Verification items for the finished model (mm, model axes). Face numbers are marked on the shaded views. A direction names the side the tool comes from. Round coordinates to 2 decimals unless told otherwise and drop trailing zeros. Order: outer loops, then holes, each group sorted by start corner. A loop starts at its lowest first (then second) coordinate and runs counter-clockwise, first axis right, second up. Notation, with made-up numbers: (33, 6.5) -> (47, 6.5) arc R32 cw to (47, 36.5) -> close; hole circle Ø9 at (2, -2). An arc over 180 degrees is marked (long way). Put each result on its own line as item: value.
from build123d import *

# Parameters (mm, degrees)
SKETCH1_W               = 35
SKETCH1_H               = 43
BOSS_EXTRUDE1_DEPTH     = 64
CUT_EXTRUDE1_DEPTH      = 77.04768241
CUT_EXTRUDE1_DEPTH_BACK = 77.04768241
CUT_EXTRUDE2_START      = -9
CUT_EXTRUDE2_DEPTH      = 9
CUT_EXTRUDE3_START      = -21
CUT_EXTRUDE3_DEPTH      = 21
SKETCH5_R               = 1.75
CUT_EXTRUDE4_DEPTH      = 21
CUT_EXTRUDE5_DEPTH      = 3
SKETCH7_R               = 1.75
CUT_EXTRUDE6_DEPTH      = 3
CUT_EXTRUDE7_DEPTH      = 2
SKETCH9_R               = 2.2
CUT_EXTRUDE8_DEPTH      = 78.474189407


# Read off the part's stored shape, not the designer's step: Cut-Extrude2, Cut-Extrude3
with BuildPart() as part:
    # Sketch1 → Boss-Extrude1 (new body)
    with BuildSketch(Plane.XY):
        Rectangle(SKETCH1_W, SKETCH1_H)
    extrude(amount=BOSS_EXTRUDE1_DEPTH)

    # Sketch2 → Cut-Extrude1 (cut, two sides: drawn at the far end of the back side and taken through both)
    with BuildSketch(Plane.ZY.offset(17.5).offset(-CUT_EXTRUDE1_DEPTH_BACK)):
        with BuildLine():
            Line((33.173885888, 11.5), (52, 11.5))
            Line((52, 11.5), (52, -10.5))
            Line((52, -10.5), (19.162446424, -10.499999995))
            add(Edge.make_bspline(
                [(19.162446424, -10.499999995), (20.832699675, -8.924322211), (23.191334331, -6.393604558), (26.156205176, -2.504954915), (28.325520723, 0.825456595), (30.873918563, 5.512287152), (32.363699443, 9.120198936), (33.173885888, 11.5)],
                knots=[0, 0, 0, 0, 0.261534973, 0.392989592, 0.556559744, 0.713681498, 1, 1, 1, 1], degree=3))
        make_face()
        with BuildLine():
            Line((0, -10.5), (0, 21.5))
            Line((0, 21.5), (24.5, 21.5))
            add(Edge.make_bspline(
                [(0, -10.5), (1.410254908, -9.794803553), (3.993077245, -8.365634948), (7.472082945, -6.021166025), (11.139491519, -3.071889035), (14.560754773, 0.394143772), (17.949614827, 4.871331165), (20.454917465, 9.23876326), (22.857889337, 14.900225374), (23.971477933, 18.909511405), (24.5, 21.5)],
                knots=[0, 0, 0, 0, 0.113112972, 0.211522862, 0.300551396, 0.450408793, 0.559434529, 0.702650577, 0.810275993, 1, 1, 1, 1], degree=3))
        make_face()
    extrude(amount=CUT_EXTRUDE1_DEPTH + CUT_EXTRUDE1_DEPTH_BACK, mode=Mode.SUBTRACT)

    # Cut-Extrude2 outline → Cut-Extrude2 (cut)
    with BuildSketch(Plane(origin=(17.5, 0, 0), x_dir=(0, 0, -1), z_dir=(1, 0, 0)).offset(CUT_EXTRUDE2_START)):
        with BuildLine():
            Line((-24.5, 21.5), (-59, 21.5))
            Line((-59, 21.5), (-59, -21.5))
            Line((-59, -21.5), (0, -21.5))
            Line((0, -21.5), (0, -10.5))
            add(Edge.make_bspline(
                [(0, -10.5), (-1.410254908, -9.794803553), (-3.993077245, -8.365634948), (-7.472082945, -6.021166025), (-11.139491519, -3.071889035), (-14.560754773, 0.394143772), (-17.949614827, 4.871331165), (-20.454917465, 9.23876326), (-22.857889337, 14.900225374), (-23.971477933, 18.909511405), (-24.5, 21.5)],
                knots=[0, 0, 0, 0, 0.113112972, 0.211522862, 0.300551396, 0.450408793, 0.559434529, 0.702650577, 0.810275993, 1, 1, 1, 1], degree=3))
        make_face()
        with BuildLine():
            Line((-52, 11.5), (-33.173885888, 11.5))
            add(Edge.make_bspline(
                [(-33.173885888, 11.5), (-32.363699443, 9.120198936), (-30.873918563, 5.512287152), (-28.325520723, 0.825456595), (-26.156205176, -2.504954915), (-23.191334331, -6.393604558), (-20.832699675, -8.924322211), (-19.162446424, -10.499999995)],
                knots=[0, 0, 0, 0, 0.286318502, 0.443440256, 0.607010408, 0.738465027, 1, 1, 1, 1], degree=3))
            Line((-19.162446424, -10.499999995), (-52, -10.5))
            Line((-52, -10.5), (-52, 11.5))
        make_face(mode=Mode.SUBTRACT)
    extrude(amount=CUT_EXTRUDE2_DEPTH, mode=Mode.SUBTRACT)

    # Cut-Extrude3 outline → Cut-Extrude3 (cut)
    with BuildSketch(Plane(origin=(8.5, 0, 0), x_dir=(0, 0, -1), z_dir=(1, 0, 0)).offset(CUT_EXTRUDE3_START)):
        with BuildLine():
            Line((-30.5, 16.5), (-59, 16.5))
            Line((-59, 16.5), (-59, -16.5))
            Line((-59, -16.5), (-51, -16.5))
            Line((-51, -16.5), (-51, -21.5))
            Line((-51, -21.5), (-10, -21.5))
            Line((-10, -21.5), (-10, -16.5))
            Line((-10, -16.5), (0, -16.5))
            Line((0, -16.5), (0, -10.5))
            add(Edge.make_bspline(
                [(0, -10.5), (-1.410254908, -9.794803553), (-3.993077245, -8.365634948), (-7.472082945, -6.021166025), (-11.139491519, -3.071889035), (-14.560754773, 0.394143772), (-17.949614827, 4.871331165), (-20.454917465, 9.23876326), (-22.857889337, 14.900225374), (-23.971477933, 18.909511405), (-24.5, 21.5)],
                knots=[0, 0, 0, 0, 0.113112972, 0.211522862, 0.300551396, 0.450408793, 0.559434529, 0.702650577, 0.810275993, 1, 1, 1, 1], degree=3))
            Line((-24.5, 21.5), (-30.5, 21.5))
            Line((-30.5, 21.5), (-30.5, 16.5))
        make_face()
        with BuildLine():
            Line((-52, 11.5), (-33.173885888, 11.5))
            add(Edge.make_bspline(
                [(-33.173885888, 11.5), (-32.363699443, 9.120198936), (-30.873918563, 5.512287152), (-28.325520723, 0.825456595), (-26.156205176, -2.504954915), (-23.191334331, -6.393604558), (-20.832699675, -8.924322211), (-19.162446424, -10.499999995)],
                knots=[0, 0, 0, 0, 0.286318502, 0.443440256, 0.607010408, 0.738465027, 1, 1, 1, 1], degree=3))
            Line((-19.162446424, -10.499999995), (-52, -10.5))
            Line((-52, -10.5), (-52, 11.5))
        make_face(mode=Mode.SUBTRACT)
    extrude(amount=CUT_EXTRUDE3_DEPTH, mode=Mode.SUBTRACT)

    # Sketch5 → Cut-Extrude4 (cut)
    with BuildSketch(Plane.XZ.offset(21.5)):
        with Locations(Location((3, 54.5, 0), (0, 0, 270))):
            Circle(SKETCH5_R)
        with Locations(Location((-7, 54.5, 0), (0, 0, 270))):
            Circle(SKETCH5_R)
        with Locations(Location((-7, 6.5, 0), (0, 0, 270))):
            Circle(SKETCH5_R)
        with Locations(Location((3, 6.5, 0), (0, 0, 270))):
            Circle(SKETCH5_R)
    extrude(amount=-CUT_EXTRUDE4_DEPTH, mode=Mode.SUBTRACT)

    # Sketch6 → Cut-Extrude5 (cut)
    with BuildSketch(Plane(origin=(0, 0, 59), x_dir=(-1, 0, 0), z_dir=(0, 0, -1))):
        Polygon((0.5, 5.095041723), (-2.7, 3.247520861), (-2.7, -0.447520861), (0.5, -2.295041723), (3.7, -0.447520861), (3.7, 3.247520861), align=None)
        Polygon((8.5, 5.095041723), (5.3, 3.247520861), (5.3, -0.447520861), (8.5, -2.295041723), (11.7, -0.447520861), (11.7, 3.247520861), align=None)
        Polygon((8.5, -6.904958277), (5.3, -8.752479139), (5.3, -12.447520861), (8.5, -14.295041723), (11.7, -12.447520861), (11.7, -8.752479139), align=None)
        Polygon((0.5, -6.904958277), (-2.7, -8.752479139), (-2.7, -12.447520861), (0.5, -14.295041723), (3.7, -12.447520861), (3.7, -8.752479139), align=None)
    extrude(amount=-CUT_EXTRUDE5_DEPTH, mode=Mode.SUBTRACT)

    # Sketch7 → Cut-Extrude6 (cut)
    with BuildSketch(Plane(origin=(0, 0, 62), x_dir=(-1, 0, 0), z_dir=(0, 0, -1))):
        with Locations((0.5, 1.4)):
            Circle(SKETCH7_R)
        with Locations((8.5, 1.4)):
            Circle(SKETCH7_R)
        with Locations((8.5, -10.6)):
            Circle(SKETCH7_R)
        with Locations((0.5, -10.6)):
            Circle(SKETCH7_R)
    extrude(amount=-CUT_EXTRUDE6_DEPTH, mode=Mode.SUBTRACT)

    # Sketch8 → Cut-Extrude7 (cut)
    with BuildSketch(Plane.XZ.offset(-16.5)):
        Polygon((1.7, 38.613804004), (1.7, 42.886195996), (-2, 45.022391992), (-5.7, 42.886195996), (-5.7, 38.613804004), (-2, 36.477608008), align=None)
    extrude(amount=-CUT_EXTRUDE7_DEPTH, mode=Mode.SUBTRACT)

    # Sketch9 → Cut-Extrude8 (cut, through all)
    with BuildSketch(Plane(origin=(0, 18.5, 0), x_dir=(-1, 0, 0), z_dir=(0, -1, 0))):
        with Locations(Location((2, -40.75, 0), (0, 0, 90))):
            Circle(SKETCH9_R)
    extrude(amount=-CUT_EXTRUDE8_DEPTH, mode=Mode.SUBTRACT)


solid = part.part
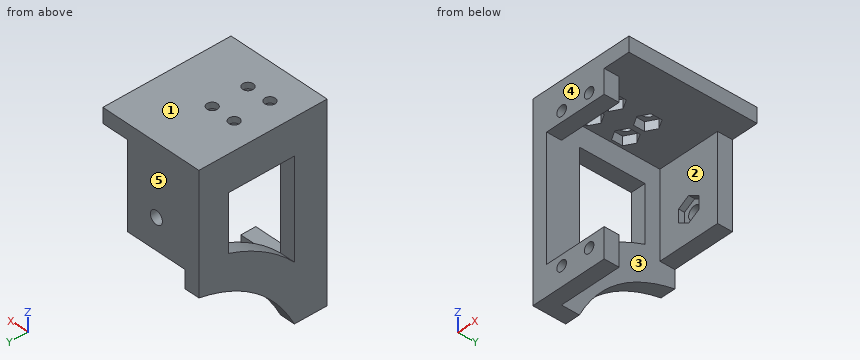
Item 1: Section check B-B on x = 4. Record the boundary of the cut face in (y, z), then the cut area to 3 significant figures.
Check sheet entries:
outline: (-21.5, 0) -> (-16.5, 0) -> (-16.5, 5.06) -> (-21.5, 5.06) -> close; (-21.5, 7.94) -> (-16.5, 7.94) -> (-16.5, 10) -> (-21.5, 10) -> close; (-21.5, 51) -> (-16.5, 51) -> (-16.5, 53.06) -> (-21.5, 53.06) -> close; (-21.5, 55.94) -> (-16.5, 55.94) -> (-16.5, 59) -> (16.5, 59) -> (16.5, 30.5) -> (21.5, 30.5) -> (21.5, 64) -> (-21.5, 64) -> close
area: 419 mm^2
Item 2: Section check D-D on y = 1.4. State how many separate pieces and enclosed holes the cut face has, then the cut area to 3 significant figures.
Check sheet entries:
separate pieces: 4
enclosed holes: 0
area: 224 mm^2
Item 3: Section check A-A on z = 54.5. Record the boundary of the cut face in (x, y), then the cut area to 3 significant figures.
Check sheet entries:
outline: (-17.5, -21.5) -> (-8.75, -21.5) -> (-8.75, -16.5) -> (-12.5, -16.5) -> (-12.5, 16.5) -> (8.5, 16.5) -> (8.5, 21.5) -> (-17.5, 21.5) -> close; (-5.25, -21.5) -> (1.25, -21.5) -> (1.25, -16.5) -> (-5.25, -16.5) -> close; (4.75, -21.5) -> (8.5, -21.5) -> (8.5, -16.5) -> (4.75, -16.5) -> close
area: 390 mm^2
Item 4: Tool access check on the marked faces 1 and 2. Record the directions out of +Z, -Z, +X, -X, +Y, -Y that give a thin tool (end or side, any length) a straight path to the whole face; none if there is none.
Check sheet entries:
face 1: +Z, +X, -X, +Y, -Y
face 2: -Z, +X
Item 5: Section check C-C on x = 12.5. Record the boundary of the cut face in (y, z).
Check sheet entries:
outline: (-21.5, 59) -> (21.5, 59) -> (21.5, 64) -> (-21.5, 64) -> close
Item 6: Gauge pin test, flat ends, axial feed: pin 1 Ø6 at (x, z) = (-3, 36.5) entering from -Y; pin 2 Ø12 at (x, y) = (-6, 1) entering from -Z; pin 3 Ø8 at (x, z) = (-2.5, 5) entering from +Y. Record the tip position at first contact, or that the pin passes through.
Check sheet entries:
pin 1: stops at y = 16.5
pin 2: stops at z = 59
pin 3: stops at y = -16.5
Item 7: Material ranges on L1, parallel to X at y = -18, z = 6.5; L2, parallel to X at y = 1.5, z = 61; L3, parallel to Y at x = -11.5, z = 54.5, recorded low to high. Write a range as [from, to].
Check sheet entries:
L1: x = [-17.5, -8.75], [-5.25, 1.25], [4.75, 8.5]
L2: x = [-17.5, -11.7], [-5.3, -3.7], [2.7, 17.5]
L3: y = [-21.5, -16.5], [16.5, 21.5]
Item 8: Release check for a two-part mould opening along Y. For the marked faces 3, 4 and 5 record: +Y half, -Y half, draft (parallel to the pull), parting line (faces both ways), or undercut.
Check sheet entries:
face 3: undercut
face 4: -Y half
face 5: +Y half
